For this review, take the finished solid that the model builds, in its own axes (mm). A direction names the side the tool comes from. Give positions to 0.01 mm unless a question says otherwise; leave off trailing zeros. Loops run counter-clockwise (first coordinate to the right, second up) from the corner with the lowest first, then second, coordinate; pieces in that order, holes last. Notation, with made-up numbers: (-9, 72) -> (0, 72) arc R21 ccw to (0, 76) -> close; hole circle Ø1 at (-12.75, -31). An arc over 180 degrees is marked (long way). Answer as CSV lines item,"result". Start each with the question number.
Item 1: The part is to be moulded in two halves that separate along X. For faces 1 (the face through (0, 5, 2)), 2 (the face through (-5, 0, 2)), 3 (the face through (4, 4, 0)), 4 (the face through (145.2, 0, 2)), say which applies: +X half, -X half, draft (parallel to the pull), parting line (faces both ways), or undercut.
Item 2: For L1, parallel to X at y = -0.5, z = -8; L2, parallel to X at y = 1.5, z = -83; L3, parallel to Z at x = 78.5, y = 0, list the stretches that pass through material, from the lowest coordinate up. Write a range as from..to.
Item 3: Clearance check with flat-ended pins moving along their axes: P1, Ø1.5, axis at y = -2.5, z = -13.5, coming from the +X side; P2, Ø2, axis at x = 18, y = -3, coming from the +Z side; P3, Ø4, axis at x = 1.5, y = 3.5, coming from the -Z side. State where each tip first meets the part, or that it passes through.
Item 4: Machinability: for faces 5 (the face through (144, 4, 0)), 6 (the face through (144, -4, 0)), 7 (the face through (136, -4, 0)), which of the approach directions +Z, -Z, +X, -X, +Y, -Y give a long, thin tool a straight path to every point of the face, cutting with its end or side? Answer none if there is none.
Item 5: Add section A-A on y = -3. State the section outline as (x, z) points.
Item 6: Add section B-B on z = -7. State the section outline as (x, y) points.
```python
from build123d import *

# Parameters (mm, degrees)
SKETCH6_R           = 5
SKETCH8_W           = 10
SKETCH8_H           = 10
BOSS_EXTRUDE1_DEPTH = 5
SKETCH9_W           = 10
SKETCH9_H           = 10
BOSS_EXTRUDE2_DEPTH = 5


with BuildPart() as part:
    # Sweep1: sweep along a path in Sketch7
    with BuildLine(Plane(origin=(0, 0, 0), x_dir=(1, 0, 0), z_dir=(0, 1, 0))) as sweep1_path:
        Line((0, 0), (0, 50))
        ThreePointArc((0, 50), (70.1, 120.1), (140.2, 50))
        Line((140.2, 50), (140.2, 0))
    # Sketch6 → Sweep1 (sweep)
    with BuildSketch(Plane.XY):
        Circle(SKETCH6_R)
    sweep(path=sweep1_path.line)

    # Sketch8 → Boss-Extrude1 (add)
    with BuildSketch(Plane.XY):
        Rectangle(SKETCH8_W, SKETCH8_H)
    extrude(amount=BOSS_EXTRUDE1_DEPTH)

    # Sketch9 → Boss-Extrude2 (add)
    with BuildSketch(Plane.XY):
        with Locations((140.2, 0)):
            Rectangle(SKETCH9_W, SKETCH9_H)
    extrude(amount=BOSS_EXTRUDE2_DEPTH)


solid = part.part
```
Computed values:
1,face 1,"draft"
1,face 2,"-X half"
1,face 3,"undercut"
1,face 4,"+X half"
2,L1,"-4.97..4.97, 135.23..145.17"
2,L2,"2.9..13.72, 126.48..137.3"
2,L3,"-124.63..-114.56"
3,P1,"x = 144.88"
3,P2,"z = -88.98"
3,P3,"z = -82.69"
4,face 5,"-Z, +X, +Y"
4,face 6,"-Z, +X, -Y"
4,face 7,"-Y"
5,outline,"(-5, 0) -> (-4, 0) -> (-4, -50) arc R74.1 ccw to (144.2, -50) -> (144.2, 0) -> (145.2, 0) -> (145.2, 5) -> (135.2, 5) -> (135.2, 0) -> (136.2, 0) -> (136.2, -50) arc R66.1 cw to (4, -50) -> (4, 0) -> (5, 0) -> (5, 5) -> (-5, 5) -> close"
6,outline,"circle Ø10 at (0, 0); circle Ø10 at (140.2, 0)"
